```python
from build123d import *

# Parameters (mm, degrees)
BOSS_EXTRUDE1_DEPTH = 20
SKETCH2_R           = 2
CUT_EXTRUDE1_DEPTH  = 5
SKETCH3_R           = 2
CUT_EXTRUDE2_DEPTH  = 5
FILLET1_R           = 3


with BuildPart() as part:
    # Sketch1 → Boss-Extrude1 (new body)
    with BuildSketch(Plane(origin=(0, 0, 0), x_dir=(1, 0, 0), z_dir=(0, 1, 0))):
        Polygon((0, 0), (0, 30), (4, 30), (4, 4), (30, 4), (30, 0), align=None)
    extrude(amount=BOSS_EXTRUDE1_DEPTH)

    # Sketch2 → Cut-Extrude1 (cut, through all)
    with BuildSketch(Plane(origin=(4, 0, 0), x_dir=(0, 0, -1), z_dir=(1, 0, 0))):
        with Locations((13, 10)):
            Circle(SKETCH2_R)
        with Locations((21, 10)):
            Circle(SKETCH2_R)
    extrude(amount=-CUT_EXTRUDE1_DEPTH, mode=Mode.SUBTRACT)

    # Sketch3 → Cut-Extrude2 (cut, through all)
    with BuildSketch(Plane(origin=(0, 0, -4), x_dir=(-1, 0, 0), z_dir=(0, 0, -1))):
        with Locations((-21, 10)):
            Circle(SKETCH3_R)
        with Locations((-13, 10)):
            Circle(SKETCH3_R)
    extrude(amount=-CUT_EXTRUDE2_DEPTH, mode=Mode.SUBTRACT)

    # Fillet1
    fillet1_edges = [part.edges().sort_by_distance(p)[0] for p in [
        (0, 10, 0),
        (4, 10, -4),
        (2, 20, -30),
        (2, 0, -30),
        (30, 20, -2),
        (30, 0, -2),
    ]]
    fillet(fillet1_edges, radius=FILLET1_R)


solid = part.part
```
Design review of the part built by this model. Coordinates are the model's own, in mm. A direction names the side the tool comes from. Round coordinates to 2 decimals unless told otherwise and drop trailing zeros. Write each loop counter-clockwise with the first axis right and the second up, starting at its lowest first coordinate (ties: lowest second). Pieces come first, ordered by that corner, then holes. Notation, with made-up numbers: (76.25, 45) -> (118.25, 45) arc R15 cw to (118.25, 70) -> close; hole circle Ø1 at (63, 12.25). An arc over 180 degrees is marked (long way). Answer in a Markdown table with one row per item.
Q1. Take a section at B-B, the plane z = -21. State the section outline as (x, y) points, then the cut area to 3 significant figures.
The answers:
| item | result |
|---|---|
| outline | (0, 0) -> (4, 0) -> (4, 8) -> (0, 8) -> close; (0, 12) -> (4, 12) -> (4, 20) -> (0, 20) -> close |
| area | 64.0 mm² |
Q2. Take a section at C-C, the plane x = 21. State the section outline as (y, z) points, then the cut area to 3 significant figures.
The answers:
| item | result |
|---|---|
| outline | (0, -4) -> (8, -4) -> (8, 0) -> (0, 0) -> close; (12, -4) -> (20, -4) -> (20, 0) -> (12, 0) -> close |
| area | 64.0 mm² |
Q3. Take a section at A-A, the plane y = 10. State the section outline as (x, z) points.
The answers:
| item | result |
|---|---|
| outline | (0, -30) -> (4, -30) -> (4, -23) -> (0, -23) -> close; (0, -19) -> (4, -19) -> (4, -15) -> (0, -15) -> close; (0, -11) -> (4, -11) -> (4, -7) arc R3 cw to (7, -4) -> (11, -4) -> (11, 0) -> (3, 0) arc R3 ccw to (0, -3) -> close; (15, -4) -> (19, -4) -> (19, 0) -> (15, 0) -> close; (23, -4) -> (30, -4) -> (30, 0) -> (23, 0) -> close |
Q4. Clearance check with flat-ended pins moving along their axes: pin 1 Ø8 at (y, z) = (7.5, -13) entering from +X; pin 2 Ø8 at (x, y) = (16.5, 10.5) entering from -Z. State where each tip first meets the part, or that it passes through.
The answers:
| item | result |
|---|---|
| pin 1 | x = 4 |
| pin 2 | z = -4 |
Q5. Take a section at D-D, the plane y = 16. State the section outline as (x, z) points.
The answers:
| item | result |
|---|---|
| outline | (0, -30) -> (4, -30) -> (4, -7) arc R3 cw to (7, -4) -> (30, -4) -> (30, 0) -> (3, 0) arc R3 ccw to (0, -3) -> close |
Q6. Draft analysis for pull direction Z (two halves, no side actions). For faces 1 (the face through (0.86, 10.14, -0.9)), 2 (the face through (4.86, 10.14, -4.9)), 3 (the face through (2.028, 11.352, -11.526)), state which applies: +Z half, -Z half, draft (parallel to the pull), parting line (faces both ways), or undercut.
The answers:
| item | result |
|---|---|
| face 1 | +Z half |
| face 2 | -Z half |
| face 3 | undercut |
Q7. To check wall thickness, follow L1, parallel to Y at x = 13, z = -3; L2, parallel to X at y = 9.75, z = -3.25; L3, parallel to Z at x = 15.75, y = 7.5. State the ranges of each line that lie inside material, in increasing order. Write a range as [from, to].
The answers:
| item | result |
|---|---|
| L1 | [0, 8], [12, 20] |
| L2 | [0, 11.02], [14.98, 19.02], [22.98, 30] |
| L3 | [-4, 0] |
Q8. For faces 4 (the face through (4, 9.9, -18.7)), 5 (the face through (2.03, 0.86, -29.1)), list the 3-axis set-ups (+Z, -Z, +X, -X, +Y, -Y) from which the entire face can be reached by the end or side of a thin tool; tool diameter is ignored.
The answers:
| item | result |
|---|---|
| face 4 | -Z, +X, +Y, -Y |
| face 5 | -Z, +X, -X, -Y |
